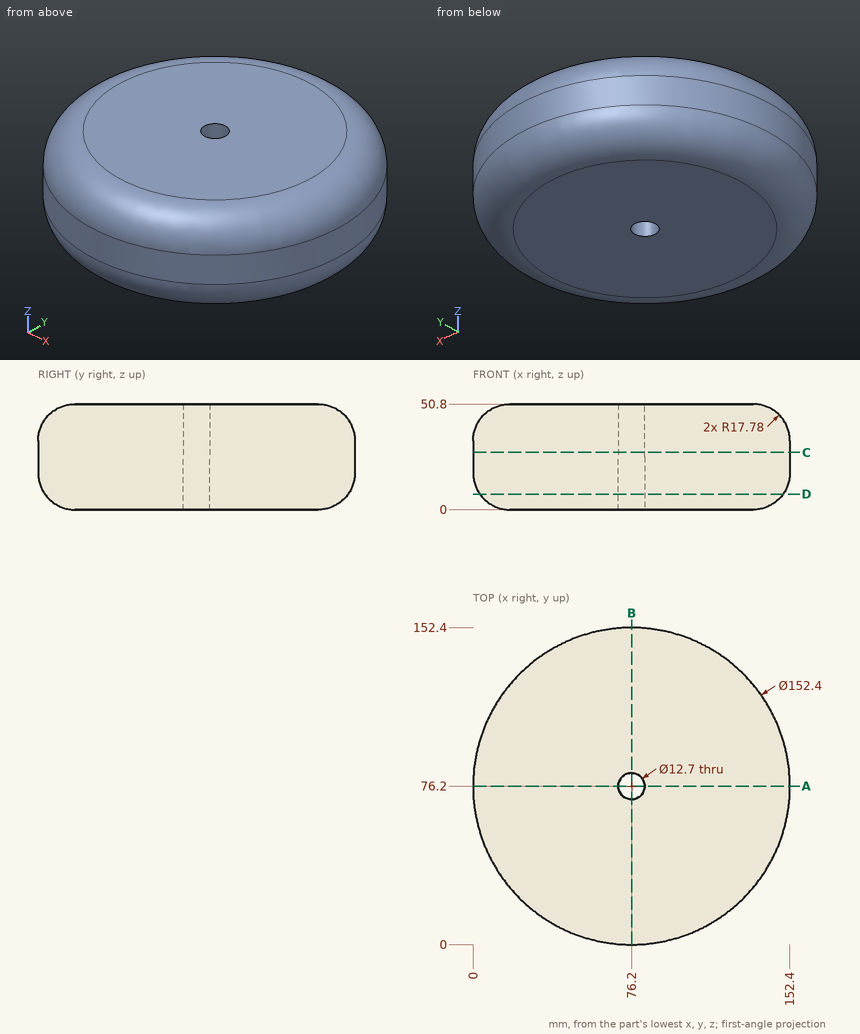
The drawing under review shows one solid part. Ordinate dimensions are in mm from its lowest x, y, z. Round coordinates to 2 decimals unless told otherwise and drop trailing zeros. Order: outer loops, then holes, each group sorted by start corner. A loop starts at its lowest first (then second) coordinate and runs counter-clockwise, first axis right, second up. Notation, with made-up numbers: M 24.25,73.25 L 41.25,73.25 A13 ccw 41.25,96.25 Z; hole C -8.5,-1 d7. An arc over 180 degrees is marked long. Answer as CSV lines item,"result". Start each with the question number.
1) Add section D-D (z = 7.5). Give the boundary of the cut face in (x, y).
2) Wall thickness on line 1 along X through (y, z) = (76.2, 32.25); line 2 along X through (y, z) = (76.2, 39.25); line 3 along Y through (x, z) = (76.2, 45): over which ranges is each line inside the solid? List them lowest first. Write a range as [from, to].
3) Add section A-A (y = 76.2). Give the boundary of the cut face in (x, z).
4) Add section C-C (z = 27.5). Give the boundary of the cut face in (x, y).
5) For pin 1 Ø2 at (x, z) = (78.5, 15.5) entering from -Y; pin 2 Ø5 at (x, z) = (111.5, 33) entering from +Y; pin 3 Ø7.5 at (x, y) = (76.2, 76.2) entering from -Z; pin 4 Ø8 at (x, z) = (105.5, 34.5) entering from +Y, all flat-tipped, find the tip position at first contact; note any pin that passes through.
Resolved:
1,outline,"C 76.2,76.2 d145.85; hole C 76.2,76.2 d12.7"
2,line 1,"[0, 69.85], [82.55, 152.4]"
2,line 2,"[1.13, 69.85], [82.55, 151.27]"
2,line 3,"[4.64, 69.85], [82.55, 147.76]"
3,outline,"M 0,17.78 A17.78 ccw 17.78,0 L 69.85,0 L 69.85,50.8 L 17.78,50.8 A17.78 ccw 0,33.02 Z; M 82.55,0 L 134.62,0 A17.78 ccw 152.4,17.78 L 152.4,33.02 A17.78 ccw 134.62,50.8 L 82.55,50.8 Z"
4,outline,"C 76.2,76.2 d152.4; hole C 76.2,76.2 d12.7"
5,pin 1,"y = 0.08"
5,pin 2,"y = 144.98"
5,pin 3,"through"
5,pin 4,"y = 148.04"
